```python
from build123d import *

# Parameters (mm, degrees)
BOSS_EXTRUDE1_DEPTH = 0.6096
SKETCH5_R           = 2.25
CUT_EXTRUDE2_DEPTH  = 0.6096
SKETCH6_R           = 1.25
CUT_EXTRUDE5_DEPTH  = 0.6096
SKETCH7_R           = 1.25
CUT_EXTRUDE6_DEPTH  = 0.6096


with BuildPart() as part:
    # Sketch1 → Boss-Extrude1 (new body)
    with BuildSketch(Plane(origin=(16.997226787, -4.149929847, 204.631375634), x_dir=(0.9965694099183702, 0.001959509651517015, -0.0827379691367708), z_dir=(-0.08276069418699705, 0.02020630066742911, -0.9963645783100802))):
        Polygon((-405.631572024, 283.216979703), (-385.692572024, 283.216979703), (-385.692572024, 323.856979703), (-405.014358213, 323.856979703), (-432.414358217, 323.856979703), (-445.097076418, 323.856979703), (-465.359895626, 323.856979703), (-479.498480719, 323.856979703), (-500.373572024, 323.856979703), (-520.312572024, 323.856979703), (-520.312572024, 283.216979703), (-500.373572024, 283.216979703), (-500.373572024, 250.003685703), (-479.037572024, 250.003685703), (-479.037572024, 283.216979703), (-426.967572024, 283.216979703), (-426.967572024, 250.003685703), (-405.631572024, 250.003685703), align=None)
    extrude(amount=BOSS_EXTRUDE1_DEPTH)

    # Sketch5 → Cut-Extrude2 (cut)
    with BuildSketch(Plane(origin=(16.946775868, -4.137612086, 204.023991787), x_dir=(-0.9965694494101686, -0.0016780440853138524, 0.08274368054637986), z_dir=(-0.08276069418699686, 0.020206300667429084, -0.9963645783100801))):
        with Locations(Location((461.99617795, -318.987055127, 0), (0, 0, 0.096164523))):
            Circle(SKETCH5_R)
        with Locations(Location((452.956635294, -318.984510283, 0), (0, 0, 0.096164523))):
            Circle(SKETCH5_R)
        with Locations(Location((443.917092638, -318.981965439, 0), (0, 0, 0.096164523))):
            Circle(SKETCH5_R)
    cut_extrude2 = extrude(amount=-CUT_EXTRUDE2_DEPTH, mode=Mode.SUBTRACT)

    # Mirror1: Cut-Extrude2 across plane
    add(cut_extrude2.mirror(Plane(origin=(0.085159645, -303.474424262, -6.16154314), x_dir=(5.696257509048786e-06, -0.02029915071256955, 0.9997939509958544), z_dir=(0.00028055772663953236, -0.9997939116314238, -0.02029915151179877))), mode=Mode.SUBTRACT)

    # Sketch6 → Cut-Extrude5 (cut)
    with BuildSketch(Plane(origin=(16.946775868, -4.137612086, 204.023991787), x_dir=(-0.9965694494101686, -0.0016780440853136297, 0.08274368054637984), z_dir=(-0.08276069418699684, 0.0202063006674291, -0.9963645783100802))):
        with Locations(Location((416.50680125, -256.173836565, 0), (0, 0, 0.096164523))):
            Circle(SKETCH6_R)
    extrude(amount=-CUT_EXTRUDE5_DEPTH, mode=Mode.SUBTRACT)

    # Sketch7 → Cut-Extrude6 (cut)
    with BuildSketch(Plane(origin=(16.946775868, -4.137612086, 204.023991787), x_dir=(-0.9965694494101686, -0.0016780440853141855, 0.08274368054637984), z_dir=(-0.08276069418699686, 0.020206300667429067, -0.9963645783100802))):
        with Locations(Location((489.681466673, -256.194436956, 0), (0, 0, 0.096164523))):
            Circle(SKETCH7_R)
    extrude(amount=-CUT_EXTRUDE6_DEPTH, mode=Mode.SUBTRACT)


solid = part.part
```
Build history of the part. All positions in model axes, mm. Round coordinates to 2 decimals unless told otherwise and drop trailing zeros. Order: outer loops, then holes, each group sorted by start corner. A loop starts at its lowest first (then second) coordinate and runs counter-clockwise, first axis right, second up. Notation, with made-up numbers: (89.5, -4.5) - (103.5, -4.5) arc R23 cw to (103.5, 26.5) - close; hole circle Ø8 at (87.5, -10.5). An arc over 180 degrees is marked (long way). Use a Markdown table: item, result.
1) Saw through at B-B on x = -425.5. Give the number of separate pieces and of enclosed holes in the cut face, and give its area (3 significant figures).
Recorded:
| item | result |
|---|---|
| separate pieces | 3 |
| enclosed holes | 0 |
| area | 19.4 mm² |
2) Flat gauge pins, fed straight in: pin 1 Ø10 at (x, y) = (-460.5, -289.5) entering from -Z; pin 2 Ø1.5 at (x, z) = (-437.5, 234) entering from -Y; pin 3 Ø4 at (y, z) = (-269, 236) entering from -X; pin 4 Ø8 at (x, y) = (-386, -309.5) entering from -Z. Where does each tip first touch, or does it go through?
Recorded:
| item | result |
|---|---|
| pin 1 | stops at z = 237.47 |
| pin 2 | passes through |
| pin 3 | stops at x = -408.48 |
| pin 4 | stops at z = 230.96 |
3) Saw through at A-A on y = -264. Write the cut outline in (x, z).
Recorded:
| item | result |
|---|---|
| outline | (-481.64, 240.17) - (-460.37, 238.4) - (-460.32, 239.01) - (-481.59, 240.78) - close; (-408.48, 234.09) - (-387.22, 232.33) - (-387.17, 232.93) - (-408.43, 234.7) - close |
4) Wall check: L1, parallel to Z at x = -391, y = -271.5; L2, parallel to Z at x = -454, y = -325. Give the ranges that are in metal, low to high.
Recorded:
| item | result |
|---|---|
| L1 | z = 232.49 to 233.1 |
| L2 | z = 236.63 to 237.25 |
5) Saw through at D-D on x = -479. Write the cut outline in (y, z), and give its area (3 significant figures).
Recorded:
| item | result |
|---|---|
| outline | (-328.92, 239.24) - (-328.9, 238.63) - (-255.07, 240.13) - (-255.08, 240.74) - close |
| area | 45.2 mm² |
6) Saw through at C-C on y = -315. Write the cut outline in (x, z), and give its area (3 significant figures).
Recorded:
| item | result |
|---|---|
| outline | (-501.49, 240.78) - (-367.34, 229.64) - (-367.29, 230.25) - (-501.44, 241.39) - close |
| area | 82.1 mm² |
